from build123d import *
from OCP.BRepFilletAPI import BRepFilletAPI_MakeChamfer

# Parameters (mm, degrees)
BOSS_EXTRUDE1_DEPTH = 300
CHAMFER1_SIZE       = 4
CHAMFER1_SIZE2      = 0.705307923
FILLET2_R           = 1.9
FILLET3_R           = 1.3
FILLET4_R           = 2.2


with BuildPart() as part:
    # Sketch1 → Boss-Extrude1 (new body)
    with BuildSketch(Plane(origin=(0, 0, 0), x_dir=(1, 0, 0), z_dir=(0, 1, 0))):
        Polygon((0, 6.443679873), (-6.128303732, 1.991206587), (-3.7875, -5.213046524), (3.7875, -5.213046524), (6.128303732, 1.991206587), align=None)
    extrude(amount=BOSS_EXTRUDE1_DEPTH)

    # Chamfer1: one chamfer whose edges measure the first distance from different faces: ONE call of the kernel's chamfer builder (chamfer() names one face for all edges)
    chamfer1_edges_1 = [part.edges().sort_by_distance(p)[0] for p in [
        (-4.957901866, 300, 1.610919968),
        (-4.957901866, 0, 1.610919968),
    ]]
    chamfer1_side_1 = [part.faces().sort_by_distance(p)[0] for p in [
        (-4.957901866, 150, 1.610919968),
    ]]
    chamfer1_edges_2 = [part.edges().sort_by_distance(p)[0] for p in [
        (0, 300, 5.213046524),
        (0, 0, 5.213046524),
    ]]
    chamfer1_side_2 = [part.faces().sort_by_distance(p)[0] for p in [
        (0, 150, 5.213046524),
    ]]
    chamfer1_edges_3 = [part.edges().sort_by_distance(p)[0] for p in [
        (4.957901866, 300, 1.610919968),
        (4.957901866, 0, 1.610919968),
    ]]
    chamfer1_side_3 = [part.faces().sort_by_distance(p)[0] for p in [
        (4.957901866, 150, 1.610919968),
    ]]
    chamfer1_edges_4 = [part.edges().sort_by_distance(p)[0] for p in [
        (-3.064151866, 0, -4.21744323),
        (-3.064151866, 300, -4.21744323),
    ]]
    chamfer1_side_4 = [part.faces().sort_by_distance(p)[0] for p in [
        (-3.064151866, 150, -4.21744323),
    ]]
    chamfer1 = BRepFilletAPI_MakeChamfer(part.part.solid().wrapped)
    for e in chamfer1_edges_1:
        chamfer1.Add(CHAMFER1_SIZE, CHAMFER1_SIZE2, e.wrapped, chamfer1_side_1[0].wrapped)  # the first distance lies on this face
    for e in chamfer1_edges_2:
        chamfer1.Add(CHAMFER1_SIZE, CHAMFER1_SIZE2, e.wrapped, chamfer1_side_2[0].wrapped)  # the first distance lies on this face
    for e in chamfer1_edges_3:
        chamfer1.Add(CHAMFER1_SIZE, CHAMFER1_SIZE2, e.wrapped, chamfer1_side_3[0].wrapped)  # the first distance lies on this face
    for e in chamfer1_edges_4:
        chamfer1.Add(CHAMFER1_SIZE, CHAMFER1_SIZE2, e.wrapped, chamfer1_side_4[0].wrapped)  # the first distance lies on this face
    add(Compound.cast(chamfer1.Shape()), mode=Mode.REPLACE)

    # Fillet2
    fillet2_edges = [part.edges().sort_by_distance(p)[0] for p in [
        (3.7875, 150, 5.213046524),
        (-6.128303732, 150, -1.991206587),
    ]]
    fillet(fillet2_edges, radius=FILLET2_R)

    # Fillet3
    fillet3_edges = [part.edges().sort_by_distance(p)[0] for p in [
        (6.128303732, 150, -1.991206587),
        (0, 150, -6.443679873),
    ]]
    fillet(fillet3_edges, radius=FILLET3_R)

    # Fillet4
    fillet4_edges = [part.edges().sort_by_distance(p)[0] for p in [
        (-3.7875, 150, 5.213046524),
    ]]
    fillet(fillet4_edges, radius=FILLET4_R)


solid = part.part
Can you work these out from the model? Positions are in its coordinate system, mm. Give positions to 0.01 mm unless a question says otherwise; leave off trailing zeros. Loops run counter-clockwise (first coordinate to the right, second up) from the corner with the lowest first, then second, coordinate; pieces in that order, holes last. Notation, with made-up numbers: (28, -2.5) - (77, -2.5) arc R31 ccw to (77, 25.5) - close; hole circle Ø2 at (20.25, 63.5). An arc over 180 degrees is marked (long way). Return JSON: item names as keys, results as strings.
1. I'm going to push flat-ended pins straight in: pin 1 Ø5 at (y, z) = (156, 1.5) entering from -X; pin 2 Ø2 at (y, z) = (72.5, -3.5) entering from +X; pin 3 Ø1.5 at (y, z) = (145, -4) entering from -X. Where does each tip first touch, or does it pass through?
Output values:
{"pin 1": "stops at x = -5.78", "pin 2": "stops at x = 5.42", "pin 3": "stops at x = -4.4"}
2. I want a section at A-A on y = 225. Please give me the cut outline in (x, z).
Output values:
{"outline": "(-5.7, -0.68) arc R1.9 ccw to (-5.01, -2.8) - (-0.76, -5.89) arc R1.3 ccw to (0.76, -5.89) - (5.36, -2.55) arc R1.3 ccw to (5.84, -1.09) - (4.21, 3.9) arc R1.9 ccw to (2.41, 5.21) - (-2.19, 5.21) arc R2.2 ccw to (-4.28, 3.69) - close"}
3. If I drill on line 1 (Z direction, x = -4, y = 180.5); line 2 (Z direction, x = -1, y = 21.5); line 3 (X direction, y = 209.5, z = -2), over which ranges is the centre line in solid material (lowest first)?
Output values:
{"line 1": "z = -3.54 to 4.26", "line 2": "z = -5.72 to 5.21", "line 3": "x = -5.65 to 5.8"}
